Verification items for this drawing (mm, ordinates from the low corner). A direction names the side the tool comes from. Coordinates: 2 decimals unless noted, no trailing zeros. Order: outer loops, then holes, each group sorted by start corner. A loop starts at its lowest first (then second) coordinate and runs counter-clockwise, first axis right, second up. Notation, with made-up numbers: (-7.75, -19) - (11.25, -19) arc R30 cw to (11.25, 8) - close; hole circle Ø3 at (23, -7.5). An arc over 180 degrees is marked (long way). One line per question, with ' | ' between items. Start each with the question number.
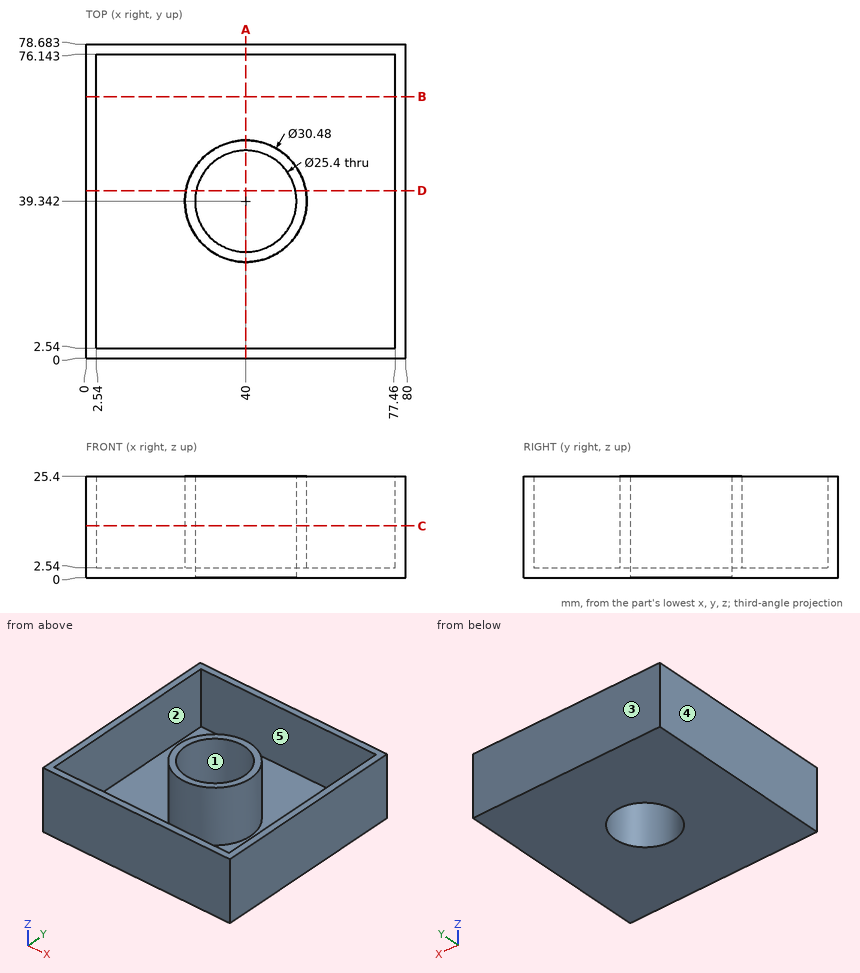
Item 1: Thickness scan on probe 1 along Y at (x, z) = (40, 9); probe 2 along Y at (x, z) = (4, 8); probe 3 along X at (y, z) = (50.5, 7.25) (1 decimal). Record the ranges inside material, lowest first. Write a range as from..to.
Item 2: Section check B-B (y = 65.5). Record the cut outline in (x, z).
Item 3: Mould release check, pull along Y, two halves, no side actions. Record for the marked faces 3, 4 and 5: +Y half, -Y half, draft (parallel to the pull), parting line (faces both ways), or undercut.
Item 4: Section check C-C (z = 13). Record the cut outline in (x, y), then the cut area to 3 significant figures.
Item 5: Set-up check for the marked faces 1 and 2: record each of +Z, -Z, +X, -X, +Y, -Y from which the full face is reachable in a straight line by a thin tool's end or side.
Item 6: Gauge pin test, flat ends, axial feed: pin 1 (11.5 mm diameter, centred on x = 23, z = 10.5, fed in from -Y); pin 2 (1.5 mm diameter, centred on x = 14, y = 25, fed in from +Z). Record the tip position at first contact, or that the pin passes through.
Item 7: Section check D-D (y = 42). Record the cut outline in (x, z).
Item 8: Section check A-A (x = 40). Record the cut outline in (y, z).
Completed:
1) probe 1: y = 0..2.54, 24.1..26.64, 52.04..54.58, 76.14..78.68 | probe 2: y = 0..2.54, 76.14..78.68 | probe 3: x = 0..2.5, 29.6..33.9, 46.1..50.4, 77.5..80
2) outline: (0, 0) - (80, 0) - (80, 25.4) - (77.46, 25.4) - (77.46, 2.54) - (2.54, 2.54) - (2.54, 25.4) - (0, 25.4) - close
3) face 3: +Y half | face 4: draft | face 5: undercut
4) outline: (0, 0) - (80, 0) - (80, 78.68) - (0, 78.68) - close; circle Ø30.48 at (40, 39.34); hole (2.54, 2.54) - (77.46, 2.54) - (77.46, 76.14) - (2.54, 76.14) - close; hole circle Ø25.4 at (40, 39.34) | area: 1,000 mm^2
5) face 1: +Z, -Z | face 2: +Z
6) pin 1: stops at y = 0 | pin 2: stops at z = 2.54
7) outline: (0, 0) - (27.58, 0) - (27.58, 25.4) - (24.99, 25.4) - (24.99, 2.54) - (2.54, 2.54) - (2.54, 25.4) - (0, 25.4) - close; (52.42, 0) - (80, 0) - (80, 25.4) - (77.46, 25.4) - (77.46, 2.54) - (55.01, 2.54) - (55.01, 25.4) - (52.42, 25.4) - close
8) outline: (0, 0) - (26.64, 0) - (26.64, 25.4) - (24.1, 25.4) - (24.1, 2.54) - (2.54, 2.54) - (2.54, 25.4) - (0, 25.4) - close; (52.04, 0) - (78.68, 0) - (78.68, 25.4) - (76.14, 25.4) - (76.14, 2.54) - (54.58, 2.54) - (54.58, 25.4) - (52.04, 25.4) - close
